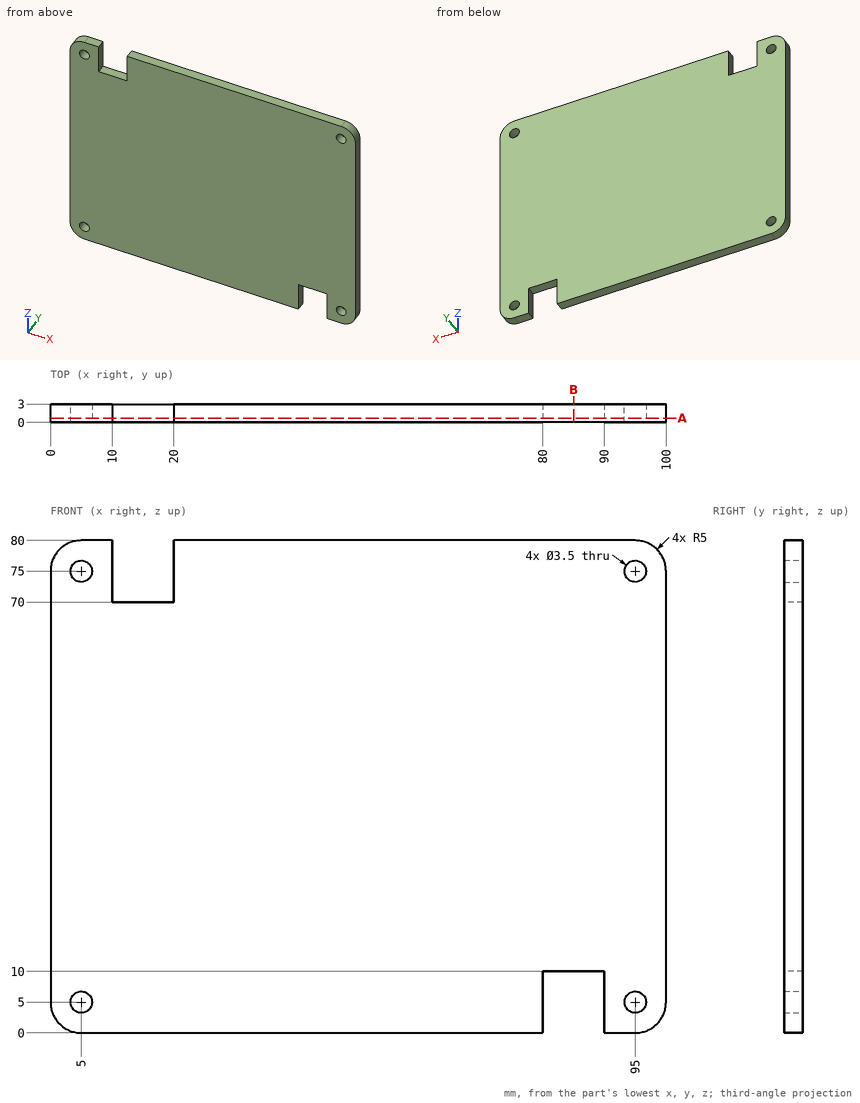
Print and shaded views of the part. All mm, measured from the part's lowest x, y and z. Coordinates: 2 decimals unless noted, no trailing zeros. Loops run counter-clockwise (first coordinate to the right, second up) from the corner with the lowest first, then second, coordinate; pieces in that order, holes last. Notation, with made-up numbers: (40, -36.75) -> (77, -36.75) arc R18 ccw to (77, -5.75) -> close; hole circle Ø7 at (-30.75, -5). An arc over 180 degrees is marked (long way). Use one line per item in the form item = value. Start each with the question number.
(1) Cut at A-A on y = 0.7. Give the cut face in (x, z), and give its area (3 significant figures).
(2) Cut at B-B on x = 85. Give the cut face in (y, z).
(3) Probe probe 1 along Z at (x, y) = (95, 1.45); probe 2 along X at (y, z) = (2.2, 75); probe 3 along X at (y, z) = (1.05, 5). List the from-to ranges inside material, lowest first. Write a range as from..to.
(4) Flat gauge pins, fed straight in: pin 1 (0.9 mm diameter, centred on x = 84.5, y = 2, fed in from -Z); pin 2 (3 mm diameter, centred on x = 95, z = 75, fed in from -Y). Where does each tip first touch, or does it go through?
Values:
q1.outline = (0, 5) arc R5 ccw to (5, 0) -> (80, 0) -> (80, 10) -> (90, 10) -> (90, 0) -> (95, 0) arc R5 ccw to (100, 5) -> (100, 75) arc R5 ccw to (95, 80) -> (20, 80) -> (20, 70) -> (10, 70) -> (10, 80) -> (5, 80) arc R5 ccw to (0, 75) -> close; hole circle Ø3.5 at (5, 5); hole circle Ø3.5 at (5, 75); hole circle Ø3.5 at (95, 5); hole circle Ø3.5 at (95, 75)
q1.area = 7,740 mm2
q2.outline = (0, 10) -> (3, 10) -> (3, 80) -> (0, 80) -> close
q3.probe_1 = 0..3.25, 6.75..73.25, 76.75..80
q3.probe_2 = 0..3.25, 6.75..10, 20..93.25, 96.75..100
q3.probe_3 = 0..3.25, 6.75..80, 90..93.25, 96.75..100
q4.pin_1 = 10
q4.pin_2 = through
